from build123d import *

# Parameters (mm, degrees)
F0_W     = 300
F0_H     = 600
F1_DEPTH = 30
F2_W     = 220
F2_H     = 520
F3_DEPTH = 35
F4_W     = 300
F4_H     = 200
F5_DEPTH = 30
F6_W     = 220
F6_H     = 120
F7_DEPTH = 40


with BuildPart() as f1:
    # F0 (on Front) → F1 (new body)
    with BuildSketch(Plane.XZ):
        with Locations((150, 300)):
            Rectangle(F0_W, F0_H)
    extrude(amount=-F1_DEPTH)

    # F2 (on face) → F3 (cut)
    with BuildSketch(Plane.XZ):
        with Locations((150, 300)):
            Rectangle(F2_W, F2_H)
    extrude(amount=-F3_DEPTH, mode=Mode.SUBTRACT)

    # F4 (on Front) → F5 (join)
    with BuildSketch(Plane.XZ):
        with Locations((-150, 100)):
            Rectangle(F4_W, F4_H)
    extrude(amount=-F5_DEPTH)

    # F6 (on face) → F7 (cut)
    with BuildSketch(Plane.XZ):
        with Locations((-150, 100)):
            Rectangle(F6_W, F6_H)
    extrude(amount=-F7_DEPTH, mode=Mode.SUBTRACT)


solid = f1.part
Geometry check sheet. Reference: the model listing, model coordinates, mm. A direction names the side the tool comes from. Round coordinates to 2 decimals unless told otherwise and drop trailing zeros. Order: outer loops, then holes, each group sorted by start corner. A loop starts at its lowest first (then second) coordinate and runs counter-clockwise, first axis right, second up. Notation, with made-up numbers: M 36,45 L 60,45 A21 ccw 60,64 Z; hole C 6,19 d10. An arc over 180 degrees is marked long. Answer in a Markdown table with one row per item. Add a question column.
Item 1: Draft check along X on faces 1 (the face through (-40, 15, 99)), 2 (the face through (21, 0, 213)), 3 (the face through (-300, 15, 99)), 4 (the face through (300, 15, 296)). Enter one of: released by +X, released by -X, zero draft, split by the parting line, or undercut.
Item 2: Sectioned sample at B-B, the plane y = 5.25. Enter the section's corners in (x, z).
Item 3: Sectioned sample at D-D, the plane z = 133. Enter the section's corners in (x, y).
Item 4: Set-up check for faces 5 (the face through (-4, 15, 0)), 6 (the face through (260, 15, 296)), 7 (the face through (0, 15, 397)): record each of +Z, -Z, +X, -X, +Y, -Y from which the full face is reachable in a straight line by a thin tool's end or side.
Item 5: Sectioned sample at C-C, the plane x = 161.5. Enter the section's corners in (y, z).
Item 6: Sectioned sample at A-A, the plane z = 524.5. Enter the section's corners in (x, y).
Item 7: Depth check by flat-ended pin: pin 1 Ø3 at (y, z) = (24.5, 278.5) entering from -X; pin 2 Ø2 at (x, y) = (-133, 4) entering from +Z. Enter the tip coordinate at first touch or a pass-through.
Item 8: Material ranges on L1, parallel to X at y = 8.5, z = 120; L2, parallel to X at y = 10.75, z = 409; L3, parallel to Z at x = 58.5, y = 24, recorded low to high. Write a range as [from, to].
Filled in:
| question | item | result |
|---|---|---|
| 1 | face 1 | undercut |
| 1 | face 2 | zero draft |
| 1 | face 3 | released by -X |
| 1 | face 4 | released by +X |
| 2 | outline | M -300,0 L 300,0 L 300,600 L 0,600 L 0,200 L -300,200 Z; hole M -260,40 L -40,40 L -40,160 L -260,160 Z; hole M 40,40 L 260,40 L 260,560 L 40,560 Z |
| 3 | outline | M -300,0 L -260,0 L -260,30 L -300,30 Z; M -40,0 L 40,0 L 40,30 L -40,30 Z; M 260,0 L 300,0 L 300,30 L 260,30 Z |
| 4 | face 5 | -Z, +X, -X, +Y, -Y |
| 4 | face 6 | +Y, -Y |
| 4 | face 7 | +Z, -X, +Y, -Y |
| 5 | outline | M 0,0 L 30,0 L 30,40 L 0,40 Z; M 0,560 L 30,560 L 30,600 L 0,600 Z |
| 6 | outline | M 0,0 L 40,0 L 40,30 L 0,30 Z; M 260,0 L 300,0 L 300,30 L 260,30 Z |
| 7 | pin 1 | stops at x = 0 |
| 7 | pin 2 | stops at z = 200 |
| 8 | L1 | x = [-300, -260], [-40, 40], [260, 300] |
| 8 | L2 | x = [0, 40], [260, 300] |
| 8 | L3 | z = [0, 40], [560, 600] |
